Build history of the part. All positions in model axes, mm. A direction names the side the tool comes from. Give positions to 0.01 mm unless a question says otherwise; leave off trailing zeros. Order: outer loops, then holes, each group sorted by start corner. A loop starts at its lowest first (then second) coordinate and runs counter-clockwise, first axis right, second up. Notation, with made-up numbers: (5.25, 71) - (27.25, 71) arc R28 ccw to (27.25, 97) - close; hole circle Ø5 at (-24.75, 64.5). An arc over 180 degrees is marked (long way). Answer in a Markdown table with one row per item.
```python
from build123d import *

# Parameters (mm, degrees)
REVOLVE1_ANGLE          = 180
REVOLVE2_ANGLE          = 180
LPATTERN1_COUNT         = 6
LPATTERN1_PITCH         = 25
BOSS_EXTRUDE1_DEPTH     = 3
CUT_EXTRUDE4_DEPTH      = 77.5
CUT_EXTRUDE4_DEPTH_BACK = 77.5
SKETCH6_R               = 2.6
CUT_EXTRUDE5_DEPTH      = 8
SKETCH7_W               = 46.5
SKETCH7_H               = 12
CUT_EXTRUDE6_DEPTH      = 8


with BuildPart() as part:
    # Sketch1 → Revolve1 (revolve)
    with BuildSketch(Plane.XY):
        with BuildLine():
            Line((62.5, 14), (-62.5, 14))
            ThreePointArc((-62.5, 14), (-72.399494937, 9.899494937), (-76.5, 0))
            Line((-76.5, 0), (76.5, 0))
            ThreePointArc((76.5, 0), (72.399494937, 9.899494937), (62.5, 14))
        make_face()
    revolve(axis=Axis((-76.5, 0, 0), (1, 0, 0)), revolution_arc=REVOLVE1_ANGLE)

    # Sketch3 → Revolve2 (revolve)
    with BuildSketch(Plane.XY.offset(5)):
        with BuildLine():
            Line((-75, 0), (-50, 0))
            ThreePointArc((-50, 0), (-62.5, 12.5), (-75, 0))
        make_face()
    revolve2 = revolve(axis=Axis((-75, 0, 5), (1, 0, 0)), revolution_arc=REVOLVE2_ANGLE)

    # LPattern1: Revolve2 ×6
    with Locations(*[(i * LPATTERN1_PITCH, 0, 0) for i in range(1, LPATTERN1_COUNT)]):
        add(revolve2)

    # Sketch4 → Boss-Extrude1 (add)
    with BuildSketch(Plane(origin=(0, 0, 0), x_dir=(-1, 0, 0), z_dir=(0, 0, -1))):
        with BuildLine():
            Line((-62.5, -14), (62.5, -14))
            ThreePointArc((62.5, -14), (76.5, 0), (62.5, 14))
            Line((62.5, 14), (-62.5, 14))
            ThreePointArc((-62.5, 14), (-76.5, 0), (-62.5, -14))
        make_face()
    extrude(amount=BOSS_EXTRUDE1_DEPTH)

    # Sketch5 → Cut-Extrude4 (cut, two sides)
    with BuildSketch(Plane(origin=(0, 0, 0), x_dir=(0, 0, -1), z_dir=(1, 0, 0))) as cut_extrude4_sk:
        Polygon((0.398662505, 13.994322713), (0.398662505, 14.646589276), (3, 14.646589276), (3, 12.5), align=None)
        Polygon((3, -14), (0.398662505, -14), (3, -12.5), align=None)
    extrude(amount=CUT_EXTRUDE4_DEPTH, mode=Mode.SUBTRACT)
    extrude(cut_extrude4_sk.sketch, amount=-CUT_EXTRUDE4_DEPTH_BACK, mode=Mode.SUBTRACT)

    # Sketch6 → Cut-Extrude5 (cut)
    with BuildSketch(Plane(origin=(0, 0, -3), x_dir=(-1, 0, 0), z_dir=(0, 0, -1))):
        with Locations(Location((0, 0, 0), (0, 0, 90))):  # turned: the seam where the file's is
            Circle(SKETCH6_R)
        with Locations(Location((62.5, 0, 0), (0, 0, 90))):  # turned: the seam where the file's is
            Circle(SKETCH6_R)
        with Locations(Location((-62.5, 0, 0), (0, 0, 90))):  # turned: the seam where the file's is
            Circle(SKETCH6_R)
    extrude(amount=-CUT_EXTRUDE5_DEPTH, mode=Mode.SUBTRACT)

    # Sketch7 → Cut-Extrude6 (cut)
    with BuildSketch(Plane(origin=(0, 0, -3), x_dir=(-1, 0, 0), z_dir=(0, 0, -1))):
        with Locations((-31.25, 0)):
            Rectangle(SKETCH7_W, SKETCH7_H)
        with Locations((31.25, 0)):
            Rectangle(SKETCH7_W, SKETCH7_H)
    extrude(amount=-CUT_EXTRUDE6_DEPTH, mode=Mode.SUBTRACT)


solid = part.part
```
1. Cut at B-B on y = 8. Write the cut outline in (x, z) (3 decimals).
Check result:
| item | result |
|---|---|
| outline | (-73.989, -3) - (73.989, -3) - (73.989, 0) arc R11.489 ccw to (71.991, 6.475) arc R9.605 ccw to (55.419, 11.489) - (44.581, 11.489) arc R9.605 ccw to (30.419, 11.489) - (19.581, 11.489) arc R9.605 ccw to (5.419, 11.489) - (-5.419, 11.489) arc R9.605 ccw to (-19.581, 11.489) - (-30.419, 11.489) arc R9.605 ccw to (-44.581, 11.489) - (-55.419, 11.489) arc R9.605 ccw to (-71.991, 6.475) arc R11.489 ccw to (-73.989, 0) - close |
2. Cut at D-D on z = 1.75. Write the cut outline in (x, y).
Check result:
| item | result |
|---|---|
| outline | (-62.5, -13.89) - (62.5, -13.89) arc R13.89 ccw to (62.5, 13.89) - (-62.5, 13.89) arc R13.89 ccw to start; hole circle Ø5.2 at (-62.5, 0); hole (-54.5, -6) - (-8, -6) - (-8, 6) - (-54.5, 6) - close; hole circle Ø5.2 at (0, 0); hole (8, -6) - (54.5, -6) - (54.5, 6) - (8, 6) - close; hole circle Ø5.2 at (62.5, 0) |
3. Two-plate mould, pull along Y, no slides. Class faces 1 (the face through (0.963, 13.237, -1.718)), 2 (the face through (-54.5, 0, 1)), 3 (the face through (-76.497, -0.308, -1.479)), 4 (the face through (-31, -6, 1)): +Y half, -Y half, draft (parallel to the pull), parting line (faces both ways), or undercut.
Check result:
| item | result |
|---|---|
| face 1 | +Y half |
| face 2 | undercut |
| face 3 | parting line |
| face 4 | undercut |
4. Drop flat-ended pins along their axis: P1, Ø4, axis at x = 38, z = 3, coming from the -Y side; P2, Ø1.5, axis at y = 5.5, z = 4.5, coming from the -X side; P3, Ø6, axis at x = 20.5, y = 1.5, coming from the -Z side. Give the stop position or say it passes through.
Check result:
| item | result |
|---|---|
| P1 | stops at y = -13.96 |
| P2 | stops at x = -74.97 |
| P3 | stops at z = 5 |
5. Cut at A-A on z = 10. Write the cut outline in (x, y), and give its area (3 significant figures).
Check result:
| item | result |
|---|---|
| outline | (-56.56, -9.8) - (-43.44, -9.8) arc R11.46 ccw to (-31.56, -9.8) - (-18.44, -9.8) arc R11.46 ccw to (-6.56, -9.8) - (6.56, -9.8) arc R11.46 ccw to (18.44, -9.8) - (31.56, -9.8) arc R11.46 ccw to (43.44, -9.8) - (56.56, -9.8) arc R11.46 ccw (long way) to (56.56, 9.8) - (43.44, 9.8) arc R11.46 ccw to (31.56, 9.8) - (18.44, 9.8) arc R11.46 ccw to (6.56, 9.8) - (-6.56, 9.8) arc R11.46 ccw to (-18.44, 9.8) - (-31.56, 9.8) arc R11.46 ccw to (-43.44, 9.8) - (-56.56, 9.8) arc R11.46 ccw (long way) to start |
| area | 3,000 mm² |
6. Probe line 1 (X direction, y = 0, z = -1.25); line 2 (X direction, y = 9.5, z = 12); line 3 (Y direction, x = -15.5, z = 1). List the from-to ranges inside material, lowest first.
Check result:
| item | result |
|---|---|
| line 1 | x = -76.5 to -65.1, -59.9 to -54.5, -8 to -2.6, 2.6 to 8, 54.5 to 59.9, 65.1 to 76.5 |
| line 2 | x = -66.62 to -58.38, -41.62 to -33.38, -16.62 to -8.38, 8.38 to 16.62, 33.38 to 41.62, 58.38 to 66.62 |
| line 3 | y = -13.96 to -6, 6 to 13.96 |
7. Which spindle directions (+Z, -Z, +X, -X, +Y, -Y) get a long thin tool onto all of the face, cutting with end or side? Do faces 5 (the face through (-1, 0, 14)), 6 (the face through (-59.922, -0.338, 0.944)), 7 (the face through (76.497, 0.308, -1.479)). Say none if no direction does.
Check result:
| item | result |
|---|---|
| face 5 | +Z |
| face 6 | -Z |
| face 7 | +Z, -Z, +X |
